Verification items for the finished model (mm, model axes). Coordinates: 2 decimals unless noted, no trailing zeros. Loops run counter-clockwise (first coordinate to the right, second up) from the corner with the lowest first, then second, coordinate; pieces in that order, holes last. Notation, with made-up numbers: (1.25, 72) - (24.25, 72) arc R33 cw to (24.25, 111) - close; hole circle Ø7 at (23, -32). An arc over 180 degrees is marked (long way). One line per item, written item: value. Start each with the question number.
(1) Section check B-B (y = 1). Count the separate pieces of the cut face and the enclosed holes in it, plus the area to 3 significant figures.
(2) Thickness scan on probe 1 along Z at (x, y) = (15, 2); probe 2 along X at (y, z) = (1.5, -11.5); probe 3 along Z at (x, y) = (-37, 1.9). Record the ranges inside material, lowest first. Write a range as [from, to].
(3) Section check A-A (z = 0). Record the boundary of the cut face in (x, y) (3 decimals), plus the area to 3 significant figures.
(4) Gauge pin test, flat end, axial feed: P1, Ø1, axis at x = 19, y = 1, coming from the -Z side (3 decimals). Record the tip position at first contact, or that the pin passes through.
(5) Section check C-C (z = 18.5). Record the boundary of the cut face in (x, y) (3 decimals).
(6) Section check D-D (x = -22). Record the boundary of the cut face in (y, z) (3 decimals).
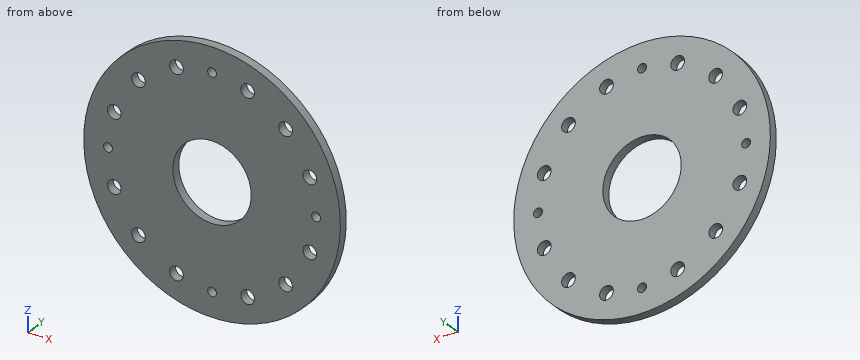
```python
from build123d import *

# Parameters (mm, degrees)
SKETCH1_R                   = 46.99
BOSS_EXTRUDE1_DEPTH         = 3.175
SKETCH2_R                   = 14.351
CUT_EXTRUDE1_DEPTH          = 3.175
CIRPATTERN1_COUNT           = 4
SKETCH5_R                   = 2.5
CUT_EXTRUDE2_DEPTH          = 5.08
CIRPATTERN2_COUNT           = 4
CIRPATTERN3_COUNT           = 2
CIRPATTERN3_ANGLE           = 25
CIRPATTERN3_COPY_1_SKETCH_R = 2.5
CIRPATTERN3_COPY_1_DEPTH    = 5.08
CIRPATTERN3_COPY_2_SKETCH_R = 2.5
CIRPATTERN3_COPY_2_DEPTH    = 5.08
CIRPATTERN3_COPY_3_SKETCH_R = 2.5
CIRPATTERN3_COPY_3_DEPTH    = 5.08
CIRPATTERN4_COUNT           = 2
CIRPATTERN4_ANGLE           = 25
CIRPATTERN4_COPY_1_SKETCH_R = 2.5
CIRPATTERN4_COPY_1_DEPTH    = 5.08
CIRPATTERN4_COPY_2_SKETCH_R = 2.5
CIRPATTERN4_COPY_2_DEPTH    = 5.08
CIRPATTERN4_COPY_3_SKETCH_R = 2.5
CIRPATTERN4_COPY_3_DEPTH    = 5.08


with BuildPart() as part:
    # Sketch1 → Boss-Extrude1 (new body)
    with BuildSketch(Plane(origin=(0, 0, 0), x_dir=(1, 0, 0), z_dir=(0, 1, 0))):
        with Locations(Location((0, 0, 0), (0, 0, 270))):
            Circle(SKETCH1_R)
    extrude(amount=BOSS_EXTRUDE1_DEPTH)

    # Sketch2 → Cut-Extrude1 (cut)
    with BuildSketch(Plane(origin=(0, 3.175, 0), x_dir=(1, 0, 0), z_dir=(0, 1, 0))):
        with Locations(Location((0, 0, 0), (0, 0, 270))):
            Circle(SKETCH2_R)
    extrude(amount=-CUT_EXTRUDE1_DEPTH, mode=Mode.SUBTRACT)

    # Sketch3 → #4 Clearance Hole1 (revolve, cut)
    with BuildSketch(Plane(origin=(0, 3.175, -38.1), x_dir=(0, 0, 1), z_dir=(1, 0, 0))):
        Polygon((0, 0), (0, 11.140574487), (1.63195, 10.16), (1.63195, 0), align=None)
    f_4_clearance_hole1 = revolve(axis=Axis((0, 9.525, -38.1), (0, -1, 0)), mode=Mode.SUBTRACT)

    # CirPattern1: #4 Clearance Hole1 ×4 about axis
    cirpattern1_axis = Axis((0, 0, 0), (0, 1, 0))
    for i in range(1, CIRPATTERN1_COUNT):
        add(f_4_clearance_hole1.rotate(cirpattern1_axis, i * 360 / CIRPATTERN1_COUNT), mode=Mode.SUBTRACT)

    # Sketch5 → Cut-Extrude2 (cut)
    with BuildSketch(Plane(origin=(0, 3.175, 0), x_dir=(1, 0, 0), z_dir=(0, 1, 0))):
        with Locations(Location((-26.940768363, 26.940768363, 0), (0, 0, 270))):
            Circle(SKETCH5_R)
    cut_extrude2 = extrude(amount=-CUT_EXTRUDE2_DEPTH, mode=Mode.SUBTRACT)

    # CirPattern2: Cut-Extrude2 ×4 about axis
    cirpattern2_axis = Axis((0, 0, 0), (0, 1, 0))
    for i in range(1, CIRPATTERN2_COUNT):
        add(cut_extrude2.rotate(cirpattern2_axis, i * 360 / CIRPATTERN2_COUNT), mode=Mode.SUBTRACT)

    # CirPattern3: Cut-Extrude2 ×2 about axis
    cirpattern3_axis = Axis((0, 0, 0), (0, 1, 0))
    for i in range(1, CIRPATTERN3_COUNT):
        add(cut_extrude2.rotate(cirpattern3_axis, i * CIRPATTERN3_ANGLE / (CIRPATTERN3_COUNT - 1)), mode=Mode.SUBTRACT)

    # CirPattern3 copy 1 sketch → CirPattern3 copy 1 (cut)
    with BuildSketch(Plane(origin=(0, 3.175, 0), x_dir=(-0.4226182617407003, 0, -0.9063077870366495), z_dir=(0, 1, 0))):
        with Locations(Location((-26.940768363, 26.940768363, 0), (0, 0, 270))):
            Circle(CIRPATTERN3_COPY_1_SKETCH_R)
    extrude(amount=-CIRPATTERN3_COPY_1_DEPTH, mode=Mode.SUBTRACT)

    # CirPattern3 copy 2 sketch → CirPattern3 copy 2 (cut)
    with BuildSketch(Plane(origin=(0, 3.175, 0), x_dir=(-0.9063077870366495, 0, 0.4226182617407002), z_dir=(0, 1, 0))):
        with Locations(Location((-26.940768363, 26.940768363, 0), (0, 0, 270))):
            Circle(CIRPATTERN3_COPY_2_SKETCH_R)
    extrude(amount=-CIRPATTERN3_COPY_2_DEPTH, mode=Mode.SUBTRACT)

    # CirPattern3 copy 3 sketch → CirPattern3 copy 3 (cut)
    with BuildSketch(Plane(origin=(0, 3.175, 0), x_dir=(0.42261826174070016, 0, 0.9063077870366496), z_dir=(0, 1, 0))):
        with Locations(Location((-26.940768363, 26.940768363, 0), (0, 0, 270))):
            Circle(CIRPATTERN3_COPY_3_SKETCH_R)
    extrude(amount=-CIRPATTERN3_COPY_3_DEPTH, mode=Mode.SUBTRACT)

    # CirPattern4: Cut-Extrude2 ×2 about axis
    cirpattern4_axis = Axis((0, 0, 0), (0, -1, 0))
    for i in range(1, CIRPATTERN4_COUNT):
        add(cut_extrude2.rotate(cirpattern4_axis, i * CIRPATTERN4_ANGLE / (CIRPATTERN4_COUNT - 1)), mode=Mode.SUBTRACT)

    # CirPattern4 copy 1 sketch → CirPattern4 copy 1 (cut)
    with BuildSketch(Plane(origin=(0, 3.175, 0), x_dir=(0.4226182617407004, 0, -0.9063077870366495), z_dir=(0, 1, 0))):
        with Locations(Location((-26.940768363, 26.940768363, 0), (0, 0, 270))):
            Circle(CIRPATTERN4_COPY_1_SKETCH_R)
    extrude(amount=-CIRPATTERN4_COPY_1_DEPTH, mode=Mode.SUBTRACT)

    # CirPattern4 copy 2 sketch → CirPattern4 copy 2 (cut)
    with BuildSketch(Plane(origin=(0, 3.175, 0), x_dir=(-0.9063077870366495, 0, -0.42261826174070044), z_dir=(0, 1, 0))):
        with Locations(Location((-26.940768363, 26.940768363, 0), (0, 0, 270))):
            Circle(CIRPATTERN4_COPY_2_SKETCH_R)
    extrude(amount=-CIRPATTERN4_COPY_2_DEPTH, mode=Mode.SUBTRACT)

    # CirPattern4 copy 3 sketch → CirPattern4 copy 3 (cut)
    with BuildSketch(Plane(origin=(0, 3.175, 0), x_dir=(-0.4226182617407005, 0, 0.9063077870366494), z_dir=(0, 1, 0))):
        with Locations(Location((-26.940768363, 26.940768363, 0), (0, 0, 270))):
            Circle(CIRPATTERN4_COPY_3_SKETCH_R)
    extrude(amount=-CIRPATTERN4_COPY_3_DEPTH, mode=Mode.SUBTRACT)


solid = part.part
```
Responses:
1. separate pieces: 1
1. enclosed holes: 17
1. area: 6,020 mm²
2. probe 1: z = [-44.53, -37.34], [-34.26, 34.26], [37.34, 44.53]
2. probe 2: x = [-45.56, -37.78], [-33.83, -8.58], [8.58, 33.83], [37.78, 45.56]
2. probe 3: z = [-28.97, -15.23], [-10.84, -1.21], [1.21, 10.84], [15.23, 28.97]
3. outline: (-46.99, 0) - (-39.732, 0) - (-39.732, 3.175) - (-46.99, 3.175) - close; (-36.468, 0) - (-14.351, 0) - (-14.351, 3.175) - (-36.468, 3.175) - close; (14.351, 0) - (36.468, 0) - (36.468, 3.175) - (14.351, 3.175) - close; (39.732, 0) - (46.99, 0) - (46.99, 3.175) - (39.732, 3.175) - close
3. area: 187 mm²
4. P1: stops at z = -43.195
5. outline: (-43.195, 0) - (43.195, 0) - (43.195, 3.175) - (-43.195, 3.175) - close
6. outline: (0, -41.522) - (3.175, -41.522) - (3.175, 41.522) - (0, 41.522) - close
